```python
from build123d import *

# Parameters (mm, degrees)
SKETCH_R      = 6
SKETCH_R_2    = 4
PAD_DEPTH     = 8
PAD001_DEPTH  = 3
FILLET_R      = 1.5
FILLET001_R   = 1
SKETCH002_W   = 2
SKETCH002_H   = 10
SKETCH002_W_2 = 10
SKETCH002_H_2 = 2
PAD002_DEPTH  = 2
CHAMFER_SIZE  = 1.99


with BuildPart() as part:
    # Sketch → Pad (new body)
    with BuildSketch(Plane.XY):
        with Locations((15, 15)):
            Circle(SKETCH_R)
        with Locations((15, 15)):
            Circle(SKETCH_R_2, mode=Mode.SUBTRACT)
    extrude(amount=PAD_DEPTH)

    # Sketch001 (on Face3 of Pad) → Pad001 (join)
    with BuildSketch(Plane(origin=(0, 0, 0), x_dir=(1, 0, 0), z_dir=(0, 0, -1))):
        with BuildLine():
            Line((0, -28.504743), (0, 0))
            Line((0, 0), (28.504743, 0))
            ThreePointArc((30.002374, -1.584264), (29.594788, -0.469562), (28.504743, 0))
            ThreePointArc((1.584264, -30.002374), (21.216341, -21.216341), (30.002374, -1.584264))
            ThreePointArc((0, -28.504743), (0.469562, -29.594788), (1.584264, -30.002374))
        make_face()
    extrude(amount=PAD001_DEPTH)

    # Fillet
    fillet_edges = [part.edges().sort_by_distance(p)[0] for p in [
        (0, 0, -1.5),
    ]]
    fillet(fillet_edges, radius=FILLET_R)

    # Fillet001
    fillet001_edges = [part.edges().sort_by_distance(p)[0] for p in [
        (0, 15.002371, -3),
        (0.43934, 0.43934, -3),
        (0.469562, 29.594788, -3),
        (15.002371, 0, -3),
        (21.216341, 21.216341, -3),
        (29.594788, 0.469562, -3),
    ]]
    fillet(fillet001_edges, radius=FILLET001_R)

    # Sketch002 (on Face4 of Fillet001) → Pad002 (join)
    with BuildSketch(Plane.XY):
        with Locations((6, 15)):
            Rectangle(SKETCH002_W, SKETCH002_H)
        with Locations((15, 6)):
            Rectangle(SKETCH002_W_2, SKETCH002_H_2)
    extrude(amount=PAD002_DEPTH)

    # Chamfer
    chamfer_edges = [part.edges().sort_by_distance(p)[0] for p in [
        (5, 15, 0),
        (15, 5, 0),
    ]]
    chamfer(chamfer_edges, length=CHAMFER_SIZE)


solid = part.part
```
Check sheet for the modelled part. Datum: model origin and axes. Units: mm. A direction names the side the tool comes from. Round coordinates to 2 decimals unless told otherwise and drop trailing zeros. Order: outer loops, then holes, each group sorted by start corner. A loop starts at its lowest first (then second) coordinate and runs counter-clockwise, first axis right, second up.
1) Scan lines: line 1 (Z direction, x = 16, y = 6.5); line 2 (Z direction, x = 9.5, y = 21); line 3 (Y direction, x = 15, z = 3.25). Record each from-to range of solid material in increasing order.
2) Section check C-C (z = -1.5). Record the boundary of the cut face in (x, y).
3) Section check A-A (z = 0.75). Record the boundary of the cut face in (x, y), and give its area (3 significant figures).
4) Section check B-B (z = 6). Record the boundary of the cut face in (x, y), and give its area (3 significant figures).
5) Tool access check on faces 1 (the flat face through (15, 7, 1)), 2 (the flat face through (6, 15, 2)), 3 (the cylindrical face through (12.05, 17.7, 3.94)), 4 (the flat face through (15, 6, 2)), 5 (the flat face through (5, 10, 1)). Record the directions out of +Z, -Z, +X, -X, +Y, -Y that give a thin tool (end or side, any length) a straight path to the whole face; none if there is none.
6) Go/stop test with flat-tipped pins: pin 1 Ø1.6 at (y, z) = (5.5, 1) entering from +X; pin 2 Ø0.6 at (x, y) = (6, 14.5) entering from +Z; pin 3 Ø1 at (y, z) = (20, 6) entering from -X; pin 4 Ø2 at (y, z) = (24.5, 2.5) entering from -X. Record where each tip stops, or that it passes through.
7) Mould release check, pull along X, two halves, no side actions. Record for faces 6 (the flat face through (10, 5, 1)), 7 (the cylindrical face through (15.191, 0.285, -2.699)), 8 (the flat face through (7, 15, 1)): +X half, -X half, draft (parallel to the pull), parting line (faces both ways), or undercut.
Result:
1. line 1: z = -3 to 2
1. line 2: z = -3 to 0
1. line 3: y = 9 to 11, 19 to 21
2. outline: (0, 1.5) arc R1.5 ccw to (1.5, 0) - (28.5, 0) arc R1.5 ccw to (30, 1.58) arc R30.16 ccw to (1.58, 30) arc R1.5 ccw to (0, 28.5) - close
3. outline: (3.76, 10) - (7, 10) - (7, 20) - (3.76, 20) - close; circle Ø12 at (15, 15); (10, 3.76) - (20, 3.76) - (20, 7) - (10, 7) - close; hole circle Ø8 at (15, 15)
3. area: 128 mm2
4. outline: circle Ø12 at (15, 15); hole circle Ø8 at (15, 15)
4. area: 62.8 mm2
5. face 1: +Z, +X, -X
5. face 2: +Z, -X, +Y, -Y
5. face 3: +Z
5. face 4: +Z, +X, -X, -Y
5. face 5: +Z, -X, -Y
6. pin 1: stops at x = 20
6. pin 2: stops at z = 2
6. pin 3: stops at x = 11.03
6. pin 4: passes through
7. face 6: -X half
7. face 7: draft
7. face 8: undercut
